The drawing under review shows one solid part. Ordinate dimensions are in mm from its lowest x, y, z. A direction names the side the tool comes from. Coordinates: 2 decimals unless noted, no trailing zeros. Loops run counter-clockwise (first coordinate to the right, second up) from the corner with the lowest first, then second, coordinate; pieces in that order, holes last. Notation, with made-up numbers: M 40.5,-11.5 L 79.5,-11.5 A18 cw 79.5,18.5 Z; hole C 62.5,1 d6. An arc over 180 degrees is marked long. Answer as a JSON object with one key per item and string values. Group by question number.
1. Insertion check: pin 1 (1 mm diameter, centred on x = 77, y = 16.5, fed in from +Z); pin 2 (6 mm diameter, centred on x = 46, y = 37.5, fed in from +Z). Each pin has a flat end and moves straight along its axis. Give the tip position at first contact, or say it passes through.
2. To check wall thickness, follow probe 1 along Y at (x, z) = (74.5, 6); probe 2 along X at (y, z) = (7.5, 23.25); probe 3 along Z at (x, y) = (34, 37.5). State the ranges of each line that lie inside material, in increasing order.
3. Consider section B-B (y = 36). State the section outline as (x, z) points.
4. Draft analysis for pull direction X (two halves, no side actions). For the marked faces 3, 4, 5 and 6, state which applies: +X half, -X half, draft (parallel to the pull), parting line (faces both ways), or undercut.
5. Consider section A-A (x = 69.5). State the section outline as (y, z) points, then the cut area to 3 significant figures.
6. Machinability: for the marked faces 1 and 2, which of the approach directions +Z, -Z, +X, -X, +Y, -Y give a long, thin tool a straight path to every point of the face, cutting with its end or side? Answer none if there is none.
7. Consider section C-C (z = 23.75). State the section outline as (x, y) points.
8. Consider section D-D (x = 57). State the section outline as (y, z) points.
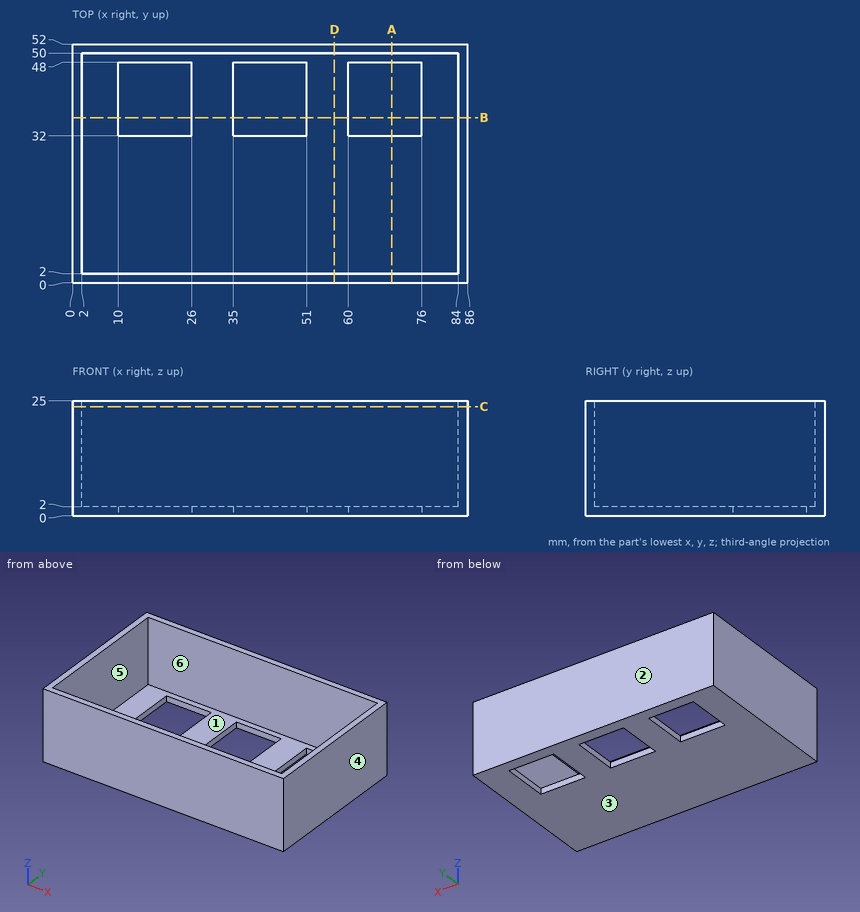
Findings below:
{
 "1": {"pin 1": "stops at z = 2", "pin 2": "passes through"},
 "2": {"probe 1": "y = 0 to 2, 50 to 52", "probe 2": "x = 0 to 2, 84 to 86", "probe 3": "z = 0 to 2"},
 "3": {"outline": "M 0,0 L 10,0 L 10,2 L 2,2 L 2,25 L 0,25 Z; M 26,0 L 35,0 L 35,2 L 26,2 Z; M 51,0 L 60,0 L 60,2 L 51,2 Z; M 76,0 L 86,0 L 86,25 L 84,25 L 84,2 L 76,2 Z"},
 "4": {"face 3": "draft", "face 4": "+X half", "face 5": "undercut", "face 6": "undercut"},
 "5": {"outline": "M 0,0 L 32,0 L 32,2 L 2,2 L 2,25 L 0,25 Z; M 48,0 L 52,0 L 52,25 L 50,25 L 50,2 L 48,2 Z", "area": "164 mm^2"},
 "6": {"face 1": "+Z", "face 2": "+Z, -Z, +X, -X, +Y"},
 "7": {"outline": "M 0,0 L 86,0 L 86,52 L 0,52 Z; hole M 2,2 L 84,2 L 84,50 L 2,50 Z"},
 "8": {"outline": "M 0,0 L 52,0 L 52,25 L 50,25 L 50,2 L 2,2 L 2,25 L 0,25 Z"}
}
